Part model, mm, in its own coordinate system. A direction names the side the tool comes from. Coordinates: 2 decimals unless noted, no trailing zeros. Write each loop counter-clockwise with the first axis right and the second up, starting at its lowest first coordinate (ties: lowest second). Pieces come first, ordered by that corner, then holes. Notation, with made-up numbers: M 29.25,69 L 45.25,69 A36 cw 45.25,104 Z; hole C -12,81.25 d6. An arc over 180 degrees is marked long. Use a Markdown table: item, result. Add a question column.
Q1. Tool access for faces 1 (the cylindrical face through (4.51, 2.46, -95.72)), 2 (the cylindrical face through (20.59, 2.54, -81.18)): list every direction of +Z, -Z, +X, -X, +Y, -Y with a clear straight run to the whole face (end or side of a thin tool).
Q2. Wall check: L1, parallel to X at y = 1.3, z = -17; L2, parallel to X at y = 3.2, z = -83; L3, parallel to X at y = 1.9, z = -130. Give the ranges that are in metal, low to high. Write a range as from..to.
Q3. Slice it at B-B on z = -135. Write the cut outline in (x, y), then the cut area to 3 significant figures.
Q4. Slice it at C-C on y = 4. Count the separate pieces of the cut face and the enclosed holes in it, then the cut area to 3 significant figures.
Q5. Mould opens along Z. For faces 3 (the flat face through (30, 3, -108)), 4 (the flat face through (133, 0, -67)), 5 (the cylindrical face through (15.056, 2.535, -67.65)) say: released by +Z, released by -Z, zero draft, split by the parting line, or undercut.
Q6. Slice it at A-A on x = 185. Write the cut outline in (y, z), then the cut area to 3 significant figures.
Q7. Pin check, flat tips, straight feed: pin 1 Ø1 at (x, y) = (8, 3.5) entering from -Z; pin 2 Ø15 at (x, z) = (115.75, -52.38) entering from -Y; pin 3 Ø1.5 at (x, y) = (28.5, 1.5) entering from -Z; pin 4 Ø2 at (y, z) = (4.5, -72.5) entering from +X. Stop position of each tip, or through.
from build123d import *

# Parameters (mm, degrees)
SKETCH1_R           = 2.1
SKETCH1_R_2         = 2.5
SKETCH1_R_3         = 2
SKETCH1_R_4         = 9.5
SKETCH1_R_5         = 1.25
SKETCH1_R_6         = 11
BOSS_EXTRUDE1_DEPTH = 5
SKETCH18_R          = 2.5
CUT_EXTRUDE15_DEPTH = 483.844656179
FILLET2_R           = 40
FILLET3_R           = 40
SKETCH21_W          = 20
SKETCH21_H          = 8
BOSS_EXTRUDE3_DEPTH = 5
SKETCH20_R          = 4
CUT_EXTRUDE17_DEPTH = 279.07373123
FILLET5_R           = 1
FILLET6_R           = 3
FILLET7_R           = 4
FILLET8_R           = 3


with BuildPart() as part:
    # Sketch1 → Boss-Extrude1 (new body)
    with BuildSketch(Plane(origin=(0, 0, 0), x_dir=(1, 0, 0), z_dir=(0, 1, 0))):
        with BuildLine():
            Line((0, 85), (0, 0))
            Line((0, 0), (220, 0))
            Line((220, 0), (220, 46))
            Line((220, 46), (210, 70))
            Line((210, 70), (210, 130))
            ThreePointArc((210, 130), (170, 170), (130, 130))
            Line((130, 130), (130, 110))
            ThreePointArc((130, 110), (127.071067812, 102.928932188), (120, 100))
            Line((120, 100), (15, 100))
            ThreePointArc((15, 100), (4.393398282, 95.606601718), (0, 85))
        make_face()
        with BuildLine():
            ThreePointArc((7.358874503, 46.014988345), (9.994913472, 52.378949376), (7.358874503, 58.742910407))
            Line((7.358874503, 58.742910407), (16.298524283, 67.682560186))
            Line((16.298524283, 67.682560186), (11.09053907, 72.890545399))
            Line((11.09053907, 72.890545399), (20.624322085, 82.424328414))
            Line((20.624322085, 82.424328414), (25.832307298, 77.216343201))
            Line((25.832307298, 77.216343201), (34.936038969, 86.320074873))
            ThreePointArc((34.936038969, 86.320074873), (41.3, 83.684035903), (47.663961031, 86.320074873))
            Line((47.663961031, 86.320074873), (75.241125497, 58.742910407))
            ThreePointArc((75.241125497, 58.742910407), (72.605086528, 52.378949376), (75.241125497, 46.014988345))
            Line((75.241125497, 46.014988345), (47.663961031, 18.437823879))
            ThreePointArc((47.663961031, 18.437823879), (41.3, 21.073862848), (34.936038969, 18.437823879))
            Line((34.936038969, 18.437823879), (7.358874503, 46.014988345))
        make_face(mode=Mode.SUBTRACT)
        with Locations(Location((95.75, 52.378949376, 0), (0, 0, 270))):
            Circle(SKETCH1_R, mode=Mode.SUBTRACT)
        with BuildLine():
            ThreePointArc((77.543356768, 70.375048681), (73.293969574, 66.641055044), (69.559975938, 70.890442238))
            ThreePointArc((69.559975938, 70.890442238), (69.148853816, 78.646273201), (66.944221963, 86.093523278))
            ThreePointArc((66.944221963, 86.093523278), (69.043291634, 91.346513523), (74.296281879, 89.247443853))
            ThreePointArc((74.296281879, 89.247443853), (77.033008956, 80.00277522), (77.543356768, 70.375048681))
        make_face(mode=Mode.SUBTRACT)
        with Locations(Location((115.75, 32.378949376, 0), (0, 0, 270))):
            Circle(SKETCH1_R, mode=Mode.SUBTRACT)
        with Locations(Location((185, 22, 0), (0, 0, 270))):
            Circle(SKETCH1_R_2, mode=Mode.SUBTRACT)
        with Locations(Location((178.187043017, 35.611788831, 0), (0, 0, 270))):
            Circle(SKETCH1_R_3, mode=Mode.SUBTRACT)
        with Locations(Location((115.75, 52.378949376, 0), (0, 0, 270))):
            Circle(SKETCH1_R_4, mode=Mode.SUBTRACT)
        with Locations(Location((135.75, 52.378949376, 0), (0, 0, 270))):
            Circle(SKETCH1_R, mode=Mode.SUBTRACT)
        with Locations(Location((115.75, 72.378949376, 0), (0, 0, 270))):
            Circle(SKETCH1_R, mode=Mode.SUBTRACT)
        with Locations(Location((127.63485968, 84.474011316, 0), (0, 0, 270))):
            Circle(SKETCH1_R_5, mode=Mode.SUBTRACT)
        with BuildLine():
            ThreePointArc((157.94568485, 75.987049461), (159.277720174, 81.48483828), (164.775508993, 80.152802956))
            ThreePointArc((164.775508993, 80.152802956), (168.201540304, 66.369956658), (163.138904601, 53.100658923))
            ThreePointArc((163.138904601, 53.100658923), (157.520629535, 52.441124786), (156.861095398, 58.059399852))
            ThreePointArc((156.861095398, 58.059399852), (160.216140338, 66.853058501), (157.94568485, 75.987049461))
        make_face(mode=Mode.SUBTRACT)
        with Locations(Location((197.592337166, 48, 0), (0, 0, 270))):
            Circle(SKETCH1_R_3, mode=Mode.SUBTRACT)
        with Locations(Location((200, 70, 0), (0, 0, 270))):
            Circle(SKETCH1_R_2, mode=Mode.SUBTRACT)
        with Locations(Location((9.83558927, 89.725342507, 0), (0, 0, 270))):
            Circle(SKETCH1_R_2, mode=Mode.SUBTRACT)
        with Locations(Location((84.83558927, 89.725342507, 0), (0, 0, 270))):
            Circle(SKETCH1_R_2, mode=Mode.SUBTRACT)
        with Locations(Location((105.63485968, 94.474011316, 0), (0, 0, 270))):
            Circle(SKETCH1_R_5, mode=Mode.SUBTRACT)
        with Locations(Location((140, 85, 0), (0, 0, 270))):
            Circle(SKETCH1_R_2, mode=Mode.SUBTRACT)
        with Locations(Location((170, 105, 0), (0, 0, 270))):
            Circle(SKETCH1_R, mode=Mode.SUBTRACT)
        with Locations(Location((145, 130, 0), (0, 0, 270))):
            Circle(SKETCH1_R, mode=Mode.SUBTRACT)
        with Locations(Location((170, 130, 0), (0, 0, 270))):
            Circle(SKETCH1_R_6, mode=Mode.SUBTRACT)
        with Locations(Location((195, 130, 0), (0, 0, 270))):
            Circle(SKETCH1_R, mode=Mode.SUBTRACT)
        with Locations(Location((170, 155, 0), (0, 0, 270))):
            Circle(SKETCH1_R, mode=Mode.SUBTRACT)
    extrude(amount=BOSS_EXTRUDE1_DEPTH)

    # Sketch18 → Cut-Extrude15 (cut, through all)
    with BuildSketch(Plane(origin=(300.638016231, 0, 207.797227621), x_dir=(-1, 0, 0), z_dir=(0, -1, 0))):
        with Locations(Location((292.118016257, 224.797227621, 0), (0, 0, 90))):
            Circle(SKETCH18_R)
        with Locations(Location((224.458016257, 224.797227621, 0), (0, 0, 90))):
            Circle(SKETCH18_R)
        with Locations(Location((156.798016257, 224.797227621, 0), (0, 0, 90))):
            Circle(SKETCH18_R)
        with Locations(Location((89.138016257, 224.797227621, 0), (0, 0, 90))):
            Circle(SKETCH18_R)
        with BuildLine():
            Line((293.118016257, 229.697227621), (291.118016257, 229.697227621))
            ThreePointArc((291.118016257, 229.697227621), (289.668016257, 231.147227621), (291.118016257, 232.597227621))
            Line((291.118016257, 232.597227621), (293.118016257, 232.597227621))
            ThreePointArc((293.118016257, 232.597227621), (294.568016257, 231.147227621), (293.118016257, 229.697227621))
        make_face()
        with BuildLine():
            Line((293.118016257, 213.347227621), (291.118016257, 213.347227621))
            ThreePointArc((291.118016257, 213.347227621), (289.668016257, 214.797227621), (291.118016257, 216.247227621))
            Line((291.118016257, 216.247227621), (293.118016257, 216.247227621))
            ThreePointArc((293.118016257, 216.247227621), (294.568016257, 214.797227621), (293.118016257, 213.347227621))
        make_face()
        with BuildLine():
            Line((225.458016257, 229.347227621), (223.458016257, 229.347227621))
            ThreePointArc((223.458016257, 229.347227621), (222.008016257, 230.797227621), (223.458016257, 232.247227621))
            Line((223.458016257, 232.247227621), (225.458016257, 232.247227621))
            ThreePointArc((225.458016257, 232.247227621), (226.908016257, 230.797227621), (225.458016257, 229.347227621))
        make_face()
        with BuildLine():
            Line((225.458016257, 213.347227621), (223.458016257, 213.347227621))
            ThreePointArc((223.458016257, 213.347227621), (222.008016257, 214.797227621), (223.458016257, 216.247227621))
            Line((223.458016257, 216.247227621), (225.458016257, 216.247227621))
            ThreePointArc((225.458016257, 216.247227621), (226.908016257, 214.797227621), (225.458016257, 213.347227621))
        make_face()
        with BuildLine():
            Line((157.798016257, 229.347227621), (155.798016257, 229.347227621))
            ThreePointArc((155.798016257, 229.347227621), (154.348016257, 230.797227621), (155.798016257, 232.247227621))
            Line((155.798016257, 232.247227621), (157.798016257, 232.247227621))
            ThreePointArc((157.798016257, 232.247227621), (159.248016257, 230.797227621), (157.798016257, 229.347227621))
        make_face()
        with BuildLine():
            Line((157.798016257, 213.347227621), (155.798016257, 213.347227621))
            ThreePointArc((155.798016257, 213.347227621), (154.348016257, 214.797227621), (155.798016257, 216.247227621))
            Line((155.798016257, 216.247227621), (157.798016257, 216.247227621))
            ThreePointArc((157.798016257, 216.247227621), (159.248016257, 214.797227621), (157.798016257, 213.347227621))
        make_face()
        with BuildLine():
            Line((90.138016257, 229.347227621), (88.138016257, 229.347227621))
            ThreePointArc((88.138016257, 229.347227621), (86.688016257, 230.797227621), (88.138016257, 232.247227621))
            Line((88.138016257, 232.247227621), (90.138016257, 232.247227621))
            ThreePointArc((90.138016257, 232.247227621), (91.588016257, 230.797227621), (90.138016257, 229.347227621))
        make_face()
        with BuildLine():
            Line((90.138016257, 213.697227621), (88.138016257, 213.697227621))
            ThreePointArc((88.138016257, 213.697227621), (86.688016257, 215.147227621), (88.138016257, 216.597227621))
            Line((88.138016257, 216.597227621), (90.138016257, 216.597227621))
            ThreePointArc((90.138016257, 216.597227621), (91.588016257, 215.147227621), (90.138016257, 213.697227621))
        make_face()
    extrude(amount=-CUT_EXTRUDE15_DEPTH, mode=Mode.SUBTRACT)

    # Fillet2
    fillet2_edges = [part.edges().sort_by_distance(p)[0] for p in [
        (210, 2.5, -70),
    ]]
    fillet(fillet2_edges, radius=FILLET2_R)

    # Fillet3
    fillet3_edges = [part.edges().sort_by_distance(p)[0] for p in [
        (220, 2.5, -46),
    ]]
    fillet(fillet3_edges, radius=FILLET3_R)

    # Sketch21 → Boss-Extrude3 (add)
    with BuildSketch(Plane(origin=(0, 5, 0), x_dir=(1, 0, 0), z_dir=(0, 1, 0))):
        with Locations((30, 104)):
            Rectangle(SKETCH21_W, SKETCH21_H)
    extrude(amount=-BOSS_EXTRUDE3_DEPTH)

    # Sketch20 → Cut-Extrude17 (cut, through all)
    with BuildSketch(Plane(origin=(0, 0, 0), x_dir=(-1, 0, 0), z_dir=(0, -1, 0))):
        with Locations(Location((-31, 99, 0), (0, 0, 90))):
            Circle(SKETCH20_R)
    extrude(amount=-CUT_EXTRUDE17_DEPTH, mode=Mode.SUBTRACT)

    # Fillet5
    fillet5_edges = [part.edges().sort_by_distance(p)[0] for p in [
        (75.241125497, 2.5, -46.014988345),
        (75.241125497, 2.5, -58.742910407),
        (47.663961031, 2.5, -86.320074873),
        (34.936038969, 2.5, -86.320074873),
        (7.358874503, 2.5, -58.742910407),
        (7.358874503, 2.5, -46.014988345),
        (34.936038969, 2.5, -18.437823879),
        (47.663961031, 2.5, -18.437823879),
    ]]
    fillet(fillet5_edges, radius=FILLET5_R)

    # Fillet6
    fillet6_edges = [part.edges().sort_by_distance(p)[0] for p in [
        (25.832307298, 2.5, -77.216343201),
        (20.624322085, 2.5, -82.424328414),
        (11.09053907, 2.5, -72.890545399),
        (16.298524283, 2.5, -67.682560186),
    ]]
    fillet(fillet6_edges, radius=FILLET6_R)

    # Fillet7
    fillet7_edges = [part.edges().sort_by_distance(p)[0] for p in [
        (40, 2.5, -100),
        (20, 2.5, -100),
    ]]
    fillet(fillet7_edges, radius=FILLET7_R)
    fillet7_2_edges = [part.edges().sort_by_distance(p)[0] for p in [
        (40, 2.5, -108),
        (20, 2.5, -108),
    ]]
    fillet(fillet7_2_edges, radius=FILLET7_R - 0.0001)  # a hair under: the kernel refuses the full size

    # Fillet8
    fillet8_edges = [part.edges().sort_by_distance(p)[0] for p in [
        (220, 2.5, 0),
        (0, 2.5, 0),
    ]]
    fillet(fillet8_edges, radius=FILLET8_R)


solid = part.part
Recorded:
| question | item | result |
|---|---|---|
| 1 | face 1 | -Z, -X, +Y, -Y |
| 1 | face 2 | +Y, -Y |
| 2 | L1 | 0..6.02, 11.02..73.68, 78.68..141.34, 146.34..209, 214..220 |
| 2 | L2 | 0..31.62, 50.98..68.09, 76.4..138.5, 141.5..210 |
| 2 | L3 | 130..142.9, 147.1..159, 181..192.9, 197.1..210 |
| 3 | outline | M 130.31,0 L 160.2,0 L 160.2,5 L 130.31,5 Z; M 179.8,0 L 209.69,0 L 209.69,5 L 179.8,5 Z |
| 3 | area | 299 mm² |
| 4 | separate pieces | 1 |
| 4 | enclosed holes | 35 |
| 4 | area | 22,000 mm² |
| 5 | face 3 | released by -Z |
| 5 | face 4 | zero draft |
| 5 | face 5 | undercut |
| 6 | outline | M 0,-167.08 L 5,-167.08 L 5,-24.5 L 0,-24.5 Z; M 0,-19.5 L 5,-19.5 L 5,0 L 0,0 Z |
| 6 | area | 810 mm² |
| 7 | pin 1 | z = -98.52 |
| 7 | pin 2 | through |
| 7 | pin 3 | z = -108 |
| 7 | pin 4 | x = 210.53 |
